```python
from build123d import *

# Parameters (mm, degrees)
SKETCH1_R                                    = 23
MAIN_BODY_DEPTH                              = 17
SHELL1_T                                     = -2.6
SKETCH22_R                                   = 20.400000000000006
SKETCH22_R_2                                 = 17.6
SIDE_PADDING_DEPTH                           = 14.4
SKETCH24_R                                   = 2.5000000000000004
SKETCH24_R_2                                 = 2.4999999999999982
SCREW_SUPPORTS_DEPTH                         = 6.8
CSK_SLOT_FOR_M1_6_COUNTERSUNK_FLAT_H_2_COUNT = 2
CSK_SLOT_FOR_M1_6_COUNTERSUNK_FLAT_H_2_PITCH = 27.712812921102078
CSK_SLOT_FOR_M1_6_COUNTERSUNK_FLAT_H_3_COUNT = 2
CSK_SLOT_FOR_M1_6_COUNTERSUNK_FLAT_H_3_PITCH = 27.712812921101964
CONNECTOR_BODY_DEPTH                         = 6
SKETCH29_W                                   = 1.9999999999999991
SKETCH29_H                                   = 3
CONNECTOR_CUTS_DEPTH                         = 47.00572879607992
FILLET2_R                                    = 2
POGO_HOLE_DEPTH                              = 4.5
POGO_TOP_SUPPORT_DEPTH                       = 0.6
POGO_BACK_SUPPORT_DEPTH                      = 0.6
MIDDLE_WIRE_CUT_DEPTH                        = 40.83716857408418
SKETCH35_R                                   = 3.3000000000000003
SLIP_RING_HOLE_DEPTH                         = 36.57189902155914


with BuildPart() as part:
    # Sketch1 → main body (new body)
    with BuildSketch(Plane(origin=(0, 0, 0), x_dir=(1, 0, 0), z_dir=(0, 1, 0))):
        with Locations(Location((0, 0, 0), (0, 0, 270))):
            Circle(SKETCH1_R)
    extrude(amount=MAIN_BODY_DEPTH)

    # Shell1
    shell1_openings = [part.faces().sort_by_distance(p)[0] for p in [
        (0, 17, 0),
    ]]
    offset(amount=SHELL1_T, openings=shell1_openings, kind=Kind.INTERSECTION)

    # Sketch22 → side padding (add)
    with BuildSketch(Plane(origin=(0, 2.6, 0), x_dir=(1, 0, 0), z_dir=(0, 1, 0))):
        Circle(SKETCH22_R)
        with Locations(Location((0, 0, 0), (0, 0, 270))):
            Circle(SKETCH22_R_2, mode=Mode.SUBTRACT)
    extrude(amount=SIDE_PADDING_DEPTH)

    # Sketch24 → screw supports (add)
    with BuildSketch(Plane(origin=(0, 2.6, 0), x_dir=(1, 0, 0), z_dir=(0, 1, 0))):
        with Locations((-8.000000000000066, 13.856406460550984)):
            Circle(SKETCH24_R)
        with Locations((16.00000000000061, 1.09033e-12)):
            Circle(SKETCH24_R_2)
        with Locations((-7.999999999998755, -13.856406460551078)):
            Circle(SKETCH24_R)
    extrude(amount=SCREW_SUPPORTS_DEPTH)

    # Sketch26 → CSK SLOT for M1.6 Countersunk Flat Head Screw2 (revolve, cut)
    with BuildSketch(Plane(origin=(-7.999999999999872, 0, 13.856406460551092), x_dir=(0, 0, -1), z_dir=(1, 0, 0))):
        Polygon((0, 0), (-4.16e-15, 17), (0.899999999999995, 17), (0.899999999999999, 8.4), (1.799999999999998, 7.5), (1.7999999999999996, -3.47e-15), align=None)
    csk_slot_for_m1_6_countersunk_flat_head = revolve(axis=Axis((-7.999999999999872, -6.349999999999991, 13.856406460551092), (0, 1, 0)), mode=Mode.SUBTRACT)

    # CSK SLOT for M1.6 Countersunk Flat H 2: CSK SLOT for M1.6 Countersunk Flat Head Screw2 ×2
    with Locations(*[(0, 0, -i * CSK_SLOT_FOR_M1_6_COUNTERSUNK_FLAT_H_2_PITCH) for i in range(1, CSK_SLOT_FOR_M1_6_COUNTERSUNK_FLAT_H_2_COUNT)]):
        add(csk_slot_for_m1_6_countersunk_flat_head, mode=Mode.SUBTRACT)

    # CSK SLOT for M1.6 Countersunk Flat H 3: CSK SLOT for M1.6 Countersunk Flat Head Screw2 ×2
    with Locations(*[Vector(0.8660254037844364, 0, -0.5000000000000041) * (i * CSK_SLOT_FOR_M1_6_COUNTERSUNK_FLAT_H_3_PITCH) for i in range(1, CSK_SLOT_FOR_M1_6_COUNTERSUNK_FLAT_H_3_COUNT)]):
        add(csk_slot_for_m1_6_countersunk_flat_head, mode=Mode.SUBTRACT)

    # Sketch28 → connector body (add)
    with BuildSketch(Plane.XZ):
        Polygon((2.0319134377332504, -16.7026098711818), (13.309106732280016, -10.235391659506115), (0.3746703089286471, 12.318994929587399), (-10.90252298561811, 5.8517767179117195), align=None)
    extrude(amount=CONNECTOR_BODY_DEPTH)

    # Sketch29 → connector cuts (cut, through all)
    with BuildSketch(Plane(origin=(-5.223545835654305, 0, 9.108543139189257), x_dir=(0.8674764072728275, 0, 0.4974783239750529), z_dir=(-0.4974783239750529, 0, 0.8674764072728275))):
        with Locations((-5.5465493958704535, -1.5)):
            Rectangle(SKETCH29_W, SKETCH29_H)
        Polygon((6.453450604129538, 1.59e-15), (6.453450604129538, -2.9999999999999982), (4.453450604129538, -2.9999999999999987), (4.453450604129538, 1.1e-15), align=None)
    extrude(amount=-CONNECTOR_CUTS_DEPTH, mode=Mode.SUBTRACT)

    # Fillet2
    fillet2_edges = [part.edges().sort_by_distance(p)[0] for p in [
        (-10.90252298561811, -4.5, 5.8517767179117195),
        (0.3746703089286471, -4.499999999999999, 12.318994929587399),
        (-5.263926338344731, -6, 9.08538582374956),
    ]]
    fillet(fillet2_edges, radius=FILLET2_R)

    # Sketch30 → pogo hole (cut)
    with BuildSketch(Plane(origin=(-5.223545835654305, 0, 9.108543139189257), x_dir=(0.8674764072728275, 0, 0.4974783239750529), z_dir=(-0.4974783239750529, 0, 0.8674764072728275))):
        Polygon((3.953450604129541, -2.6999999999999975), (-4.046549395870457, -2.7), (-4.046549395870457, -6), (3.953450604129543, -5.999999999999997), align=None)
    extrude(amount=-POGO_HOLE_DEPTH, mode=Mode.SUBTRACT)

    # Sketch31 → pogo top support (add)
    with BuildSketch(Plane.XZ.offset(6)):
        Polygon((-6.495179509548303, 3.1918286951216346), (0.44463174863431776, 7.171655286922058), (-1.1472988880858548, 9.947579790195107), (-8.087110146268472, 5.967753198394682), align=None)
    extrude(amount=-POGO_TOP_SUPPORT_DEPTH)

    # Sketch33 → pogo back support (add)
    with BuildSketch(Plane(origin=(0, -5.4, 0), x_dir=(1, 0, 0), z_dir=(0, 1, 0))):
        Polygon((-6.4951795095483025, -3.191828695121635), (0.44463174863431776, -7.171655286922058), (-0.5503248993157871, -8.906608101467711), (-7.490136157498408, -4.926781509667289), align=None)
    extrude(amount=POGO_BACK_SUPPORT_DEPTH)

    # Sketch34 → middle wire cut (cut, through all)
    with BuildSketch(Plane.XZ.offset(6)):
        Polygon((-6.352157331722817, 6.962709846344788), (-3.1185482258849735, 1.3241131990714121), (0.35135740320633424, 3.314026494971624), (-2.8822517026315113, 8.952623142245), align=None)
    extrude(amount=-MIDDLE_WIRE_CUT_DEPTH, mode=Mode.SUBTRACT)

    # Sketch35 → slip ring hole (cut, through all)
    with BuildSketch(Plane(origin=(0, 2.6, 0), x_dir=(1, 0, 0), z_dir=(0, 1, 0))):
        Circle(SKETCH35_R)
    extrude(amount=-SLIP_RING_HOLE_DEPTH, mode=Mode.SUBTRACT)


solid = part.part
```
The model under review builds one solid part; all positions refer to its coordinate system, in mm. A direction names the side the tool comes from. Round coordinates to 2 decimals unless told otherwise and drop trailing zeros. Write each loop counter-clockwise with the first axis right and the second up, starting at its lowest first coordinate (ties: lowest second). Pieces come first, ordered by that corner, then holes. Notation, with made-up numbers: (43.25, 80) - (67.25, 80) arc R15 cw to (67.25, 87) - close; hole circle Ø7 at (-32, -17). An arc over 180 degrees is marked (long way). One line per question, with ' | ' between items.
Item 1: For faces 4 (the face through (5.02, -1.52, 0.2)), 5 (the face through (0.505, -4.188, 11.39)), 6 (the face through (-5.209, -1.528, 9.117)), 7 (the face through (15, 9.4, 1)), 8 (the face through (-0.43, -3.74, 6.67)), list the 3-axis set-ups (+Z, -Z, +X, -X, +Y, -Y) from which the entire face can be reached by the end or side of a thin tool; tool diameter is ignored.
Resolved:
face 4: +Z, +X | face 5: +Z, -Y | face 6: +Z, -X, -Y | face 7: +Y | face 8: none
Item 2: To check wall thickness, follow probe 1 along X at (y, z) = (5, 0); probe 2 along X at (y, z) = (9.15, 0); probe 3 along Y at (x, z) = (-2.5, -6). State the ranges of each line that lie inside material, in increasing order.
Resolved:
probe 1: x = -23 to -17.6, 13.5 to 14.2, 17.8 to 23 | probe 2: x = -23 to -17.6, 13.5 to 15.1, 16.9 to 23 | probe 3: y = -6 to -3, 0 to 2.6
Item 3: For P1, Ø4, axis at x = 16, z = 0, coming from the -Y side; P2, Ø4, axis at x = 4.5, z = 11.5, coming from the +Y side; P3, Ø1, axis at x = 11.5, y = 13, coming from the -Z side; P4, Ø1.1, axis at x = -8, z = -13.86, coming from the +Y side, all flat-tipped, find the tip position at first contact; note any pin that passes through.
Resolved:
P1: stops at y = 0 | P2: stops at y = 2.6 | P3: stops at z = -20.2 | P4: passes through
Item 4: Add section B-B, the plane y = 4.5. Give the boundary of the cut face in (x, z).
Resolved:
outline: circle Ø46 at (0, 0); hole (-10.48, -14.14) arc R2.5 cw (long way) to (-7, -16.15) arc R17.6 ccw to (17.48, -2.01) arc R2.5 cw (long way) to (17.48, 2.01) arc R17.6 ccw to (-7, 16.15) arc R2.5 cw (long way) to (-10.48, 14.14) arc R17.6 ccw to start; hole circle Ø3.6 at (-8, -13.86); hole circle Ø3.6 at (-8, 13.86); hole circle Ø3.6 at (16, 0)
Item 5: Add section C-C, the plane x = 10.5. Give the boundary of the cut face in (y, z).
Resolved:
outline: (-6, -11.85) - (0, -11.85) - (0, -20.46) - (17, -20.46) - (17, -14.12) - (2.6, -14.12) - (2.6, 14.12) - (17, 14.12) - (17, 20.46) - (0, 20.46) - (0, -9.36) - (-3, -9.36) - (-3, -5.34) - (-6, -5.34) - close
Item 6: Add section A-A, the plane z = 0. State how many separate pieces and enclosed holes the cut face has, then the cut area to 3 significant figures.
Resolved:
separate pieces: 3 | enclosed holes: 0 | area: 291 mm2
Item 7: The part is to be moulded in two halves that separate along Z. For faces 1 (the face through (-0.533, -5.651, 10.795)), 2 (the face through (-0.69, -3.96, 9.15)), 3 (the face through (-7, -5.4, 6)), say which applies: pulls with the +Z half, pulls with the -Z half, needs draft (parallel to the pull), parting line crosses it, or undercut.
Resolved:
face 1: pulls with the +Z half | face 2: undercut | face 3: needs draft
Item 8: Add section D-D, the plane z = -7.5. Give the boundary of the cut face in (x, y).
Resolved:
outline: (-21.74, 0) - (-0.94, 0) - (-0.94, -3) - (-3.25, -3) - (-3.25, -6) - (11.74, -6) - (11.74, -3) - (9.43, -3) - (9.43, 0) - (21.74, 0) - (21.74, 17) - (15.92, 17) - (15.92, 2.6) - (-15.92, 2.6) - (-15.92, 17) - (-21.74, 17) - close
